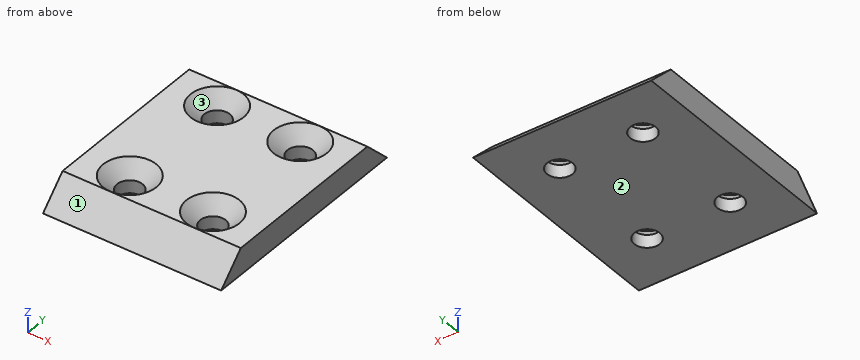
from build123d import *

# Parameters (mm, degrees)
SKETCH_1_W                   = 30
SKETCH_1_H                   = 38
EXTRUDE_1_DEPTH              = 4.5
CHAMFER_1_SIZE               = 4.5
HOLE_WIZARD_M4_1_D           = 4.3
HOLE_WIZARD_M4_1_CSINK_D     = 8.96
HOLE_WIZARD_M4_1_CSINK_ANGLE = 90


with BuildPart() as part:
    # 草图1 → 凸台-拉伸1 (new body)
    with BuildSketch(Plane.XY):
        with Locations((15, 19)):
            Rectangle(SKETCH_1_W, SKETCH_1_H)
    extrude(amount=EXTRUDE_1_DEPTH)

    # 倒角1
    chamfer_1_edges = [part.edges().sort_by_distance(p)[0] for p in [
        (15, 0, 4.5),
        (15, 38, 4.5),
    ]]
    chamfer(chamfer_1_edges, length=CHAMFER_1_SIZE - 0.0001)  # a hair under: the kernel refuses the full size

    # M4 六角凹锥坑螺钉的锥形沉头孔1 (through all)
    with Locations(Plane.XY.offset(4.5)):
        with Locations((8, 9), (8, 29), (22, 29), (22, 9)):
            CounterSinkHole(HOLE_WIZARD_M4_1_D / 2, HOLE_WIZARD_M4_1_CSINK_D / 2, counter_sink_angle=HOLE_WIZARD_M4_1_CSINK_ANGLE)


solid = part.part
Source: CAD feature listing. Evaluate the final solid. Frame: model axes, mm. Face numbers are marked on the shaded views. Coordinates: 2 decimals unless noted, no trailing zeros. Loops run counter-clockwise (first coordinate to the right, second up) from the corner with the lowest first, then second, coordinate; pieces in that order, holes last. Notation, with made-up numbers: (64.5, 66.25) - (77.5, 66.25) arc R18 cw to (77.5, 87.25) - close; hole circle Ø2 at (47, 69.25). An arc over 180 degrees is marked (long way). One line per question, with ' | ' between items.
1) Pull-direction query (Y, two-part tool) for the marked faces 1, 2 and 3; classes: released by +Y, released by -Y, zero draft, split by the parting line, or undercut.
Report:
face 1: released by -Y | face 2: zero draft | face 3: undercut
2) First-contact query: P1, Ø10, axis at x = 15, y = 24, coming from the -Z side; P2, Ø1.5, axis at x = 15, z = 3, coming from the +Y side; P3, Ø4, axis at x = 22, y = 9, coming from the +Z side; P4, Ø5.5, axis at x = 22, y = 29, coming from the +Z side. Flat tips, straight axial feed; report the tip coordinate or a pass-through.
Report:
P1: stops at z = 0 | P2: stops at y = 35.75 | P3: passes through | P4: stops at z = 2.77
3) Line query: line 1 along X through (y, z) = (29, 0.75); line 2 along Y through (x, z) = (8, 1.15); line 3 along Y through (x, z) = (23, 2). Output: solid intervals per line, ascending.
Report:
line 1: x = 0 to 5.85, 10.15 to 19.85, 24.15 to 30 | line 2: y = 1.15 to 6.85, 11.15 to 26.85, 31.15 to 36.85 | line 3: y = 2 to 7.1, 10.9 to 27.1, 30.9 to 36
4) Section D-D, the plane z = 2.6. Return loops of the section in (x, y), then the cut area to 3 significant figures.
Report:
outline: (0, 2.6) - (30, 2.6) - (30, 35.4) - (0, 35.4) - close; hole circle Ø5.16 at (8, 9); hole circle Ø5.16 at (8, 29); hole circle Ø5.16 at (22, 9); hole circle Ø5.16 at (22, 29) | area: 900 mm²
5) Section B-B, the plane x = 22. Give the number of separate pieces and of enclosed holes in the cut face, then the cut area to 3 significant figures.
Report:
separate pieces: 3 | enclosed holes: 0 | area: 101 mm²
6) Section A-A, the plane y = 9. Return loops of the section in (x, z), then the cut area to 3 significant figures.
Report:
outline: (0, 0) - (5.85, 0) - (5.85, 2.17) - (3.52, 4.5) - (0, 4.5) - close; (10.15, 0) - (19.85, 0) - (19.85, 2.17) - (17.52, 4.5) - (12.48, 4.5) - (10.15, 2.17) - close; (24.15, 0) - (30, 0) - (30, 4.5) - (26.48, 4.5) - (24.15, 2.17) - close | area: 85.4 mm²
